Geometry: final body of the model. Coordinates: model frame, mm. Coordinates: 2 decimals unless noted, no trailing zeros. Write each loop counter-clockwise with the first axis right and the second up, starting at its lowest first coordinate (ties: lowest second). Pieces come first, ordered by that corner, then holes. Notation, with made-up numbers: M 81,48.5 L 137,48.5 A10 cw 137,57.5 Z; hole C 22,26.5 d1. An arc over 180 degrees is marked long. Write item = value, one per line. Start each with the question number.
Item 1: First-contact query: pin 1 Ø3 at (x, y) = (-75.556, 50.665) entering from -Z. Flat tip, straight axial feed; report the tip coordinate or a pass-through.
Item 2: Section A-A on x = 75.56. Output: boundary loops of the cut face in (y, z) (3 decimals), plus the area to 3 significant figures.
Item 3: Ray query, L1, parallel to X at y = -34, z = 1.5; L2, parallel to Y at x = 58, z = 1.7; L3, parallel to X at y = -44.5, z = 0.7. Return the intervals inside material, ascending. Write a range as [from, to].
Solid Edge part; units mm, degrees
sketch "Sketch1" plane through (0, 0, 0) normal (0, 0, 1) x (1, 0, 0)
  line L0 (-88, -59) -> (88, -59)
  line L1 (88, -59) -> (88, 59)
  line L2 (88, 59) -> (-88, 59)
  line L3 (-88, 59) -> (-88, -59)
  dimension "D1" = 88
  dimension "D2" = 88
extrude "Protrusion1" add sketch "Sketch1" along normal blind 2
hole "Hole1" at (-9, -52.375, 0) direction (0, 0, 1) diameter 2 end up to next
hole "Hole2" at (16, -52.375, 0) direction (0, 0, 1) diameter 2 end up to next
hole "Hole3" at (0, 3, 2) direction (0, 0, -1) diameter 2 end through all
hole "Hole4" at (58, 3, 2) direction (0, 0, -1) diameter 2 end through all
hole "Hole5" at (58, -34, 2) direction (0, 0, -1) diameter 2 end through all
hole "Hole6" at (0, -34, 2) direction (0, 0, -1) diameter 2 end through all
hole "Hole7" at (-58, -34, 2) direction (0, 0, -1) diameter 2 end through all
hole "Hole8" at (-58, 3, 2) direction (0, 0, -1) diameter 2 end through all
hole "Hole9" at (-58, 40, 2) direction (0, 0, -1) diameter 2 end through all
hole "Hole10" at (58, 40, 2) direction (0, 0, -1) diameter 2 end through all
sketch "Sketch2" plane through (0, 0, 2) normal (0, 0, 1) x (1, 0, 0)
  line L0 (3.25, -59) -> (3.75, -59)
  line L1 (3.75, -58.5) -> (3.75, -59)
  line L2 (3.25, -58.5) -> (3.75, -58.5)
  line L3 (3.25, -59) -> (3.25, -58.5)
  dimension "D1" = 3.75
extrude "Cutout1" cut sketch "Sketch2" against normal through all
hole "Hole11" at (13.6, 13.665, 2) direction (0, 0, -1) diameter 3.5 end through all
hole "Hole12" at (-65.12, -44.665, 2) direction (0, 0, -1) diameter 3.5 end through all
hole "Hole13" at (13.6, -44.665, 2) direction (0, 0, -1) diameter 3.5 end through all
hole "Hole14" at (75.56, 50.665, 2) direction (0, 0, -1) diameter 3.5 end through all
hole "Hole15" at (71.6, -44.665, 2) direction (0, 0, -1) diameter 3.5 end through all
hole "Hole16" at (-75.556, 50.665, 2) direction (0, 0, -1) diameter 3.5 end through all
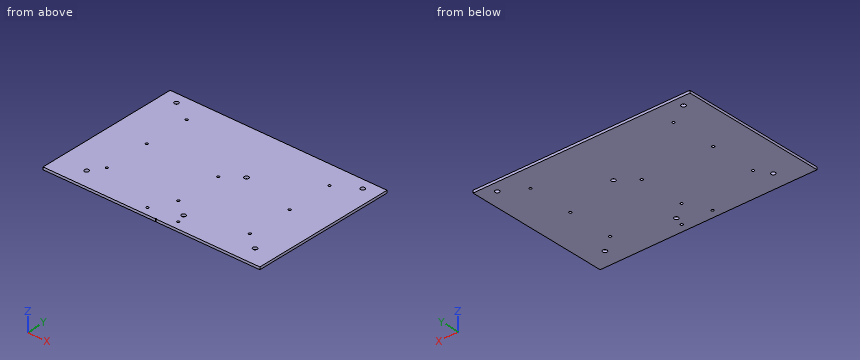
Responses:
q1.pin_1 = through
q2.outline = M -59,0 L 48.915,0 L 48.915,2 L -59,2 Z; M 52.415,0 L 59,0 L 59,2 L 52.415,2 Z
q2.area = 229 mm²
q3.L1 = [-88, -59], [-57, -1], [1, 57], [59, 88]
q3.L2 = [-59, -35], [-33, 2], [4, 39], [41, 59]
q3.L3 = [-88, -66.86], [-63.38, 11.86], [15.34, 69.86], [73.34, 88]
